Here's how the part is built. I have some questions about the finished solid (model axes, mm). A direction names the side the tool comes from. Round coordinates to 2 decimals unless told otherwise and drop trailing zeros. Order: outer loops, then holes, each group sorted by start corner. A loop starts at its lowest first (then second) coordinate and runs counter-clockwise, first axis right, second up. Notation, with made-up numbers: (-2, 23) - (37, 23) arc R6 ccw to (37, 33) - close; hole circle Ø11 at (31, 3.25). An arc over 180 degrees is marked (long way). One line per item, written item: value.
from build123d import *

# Parameters (mm, degrees)
SKETCH1_R               = 5
BOSS_EXTRUDE1_DEPTH     = 50
SKETCH2_R               = 2
CUT_EXTRUDE1_DEPTH      = 113.087037288
CUT_EXTRUDE3_DEPTH      = 10
CUT_EXTRUDE3_DEPTH_BACK = 10
SKETCH7_W               = 20
SKETCH7_H               = 39.987182744
BOSS_EXTRUDE2_REACH     = 114.087
CUT_EXTRUDE4_REACH      = 114.087
SKETCH9_W               = 20
SKETCH9_H               = 10.896319728
CUT_EXTRUDE6_REACH      = 114.087
SKETCH11_W              = 5
SKETCH11_H              = 3
SKETCH12_W              = 73
SKETCH12_H              = 70
BOSS_EXTRUDE3_DEPTH     = 3
SKETCH13_W              = 6.758772051
SKETCH13_H              = 20
CUT_EXTRUDE7_DEPTH      = 117.122297969
FILLET1_R               = 10


with BuildPart() as part:
    # Sketch1 → Boss-Extrude1 (new body)
    with BuildSketch(Plane.XY):
        with Locations((90.291740814, 26.352640412)):
            Circle(SKETCH1_R)
        Polygon((0, 3), (0, 0), (81.758772051, 0), (91.791740814, 17.924366601), (91.791740814, 23.706854983), (88.791740814, 23.706854983), (88.791740814, 18.706854983), (80, 3), align=None)
    extrude(amount=BOSS_EXTRUDE1_DEPTH)

    # Sketch2 → Cut-Extrude1 (cut, through all)
    with BuildSketch(Plane.XY):
        with Locations((90.291740814, 26.352640412)):
            Circle(SKETCH2_R)
    extrude(amount=CUT_EXTRUDE1_DEPTH, mode=Mode.SUBTRACT)

    # Sketch7 → Cut-Extrude3 (cut, two sides: drawn at the far end of the back side and taken through both)
    with BuildSketch(Plane(origin=(62.254079791, -34.846042362, 0), x_dir=(0, 0, -1), z_dir=(0.8726030546274219, -0.4884300452008377, 0)).offset(-CUT_EXTRUDE3_DEPTH_BACK)):
        with Locations((-25, 59.927032101)):
            Rectangle(SKETCH7_W, SKETCH7_H)
    extrude(amount=CUT_EXTRUDE3_DEPTH + CUT_EXTRUDE3_DEPTH_BACK, mode=Mode.SUBTRACT)

    # Sketch8 → Boss-Extrude2 (add, up to next)
    with BuildSketch(Plane.XY, mode=Mode.PRIVATE) as boss_extrude2_sk1:
        Polygon((66.951015515, 3), (66.951015515, 0), (81.758772051, 0), (79.25400484, 1.667244856), (80, 3), align=None)
    boss_extrude2_tool1 = extrude(boss_extrude2_sk1.sketch, amount=BOSS_EXTRUDE2_REACH, mode=Mode.PRIVATE) - part.part
    add(boss_extrude2_tool1.solids().sort_by_distance((73.552437, 1.463367, 0))[0])

    # Sketch9 → Cut-Extrude4 (cut, up to next)
    with BuildSketch(Plane(origin=(0, 0, 0), x_dir=(0, 0, -1), z_dir=(1, 0, 0)), mode=Mode.PRIVATE) as cut_extrude4_sk1:
        with Locations((-25, 32.01270193)):
            Rectangle(SKETCH9_W, SKETCH9_H)
    cut_extrude4_tool1 = extrude(cut_extrude4_sk1.sketch, amount=CUT_EXTRUDE4_REACH, mode=Mode.PRIVATE) & part.part
    add(cut_extrude4_tool1.solids().sort_by_distance((0, 32.012702, 25))[0], mode=Mode.SUBTRACT)

    # Sketch11 → Cut-Extrude6 (cut, up to next)
    with BuildSketch(Plane.XY.offset(50), mode=Mode.PRIVATE) as cut_extrude6_sk1:
        with Locations((2.5, 1.5)):
            Rectangle(SKETCH11_W, SKETCH11_H)
    cut_extrude6_tool1 = extrude(cut_extrude6_sk1.sketch, amount=-CUT_EXTRUDE6_REACH, mode=Mode.PRIVATE) & part.part
    add(cut_extrude6_tool1.solids().sort_by_distance((2.5, 1.5, 50))[0], mode=Mode.SUBTRACT)

    # Sketch12 → Boss-Extrude3 (add, through all)
    with BuildSketch(Plane(origin=(0, 3, 0), x_dir=(1, 0, 0), z_dir=(0, 1, 0))):
        with Locations((38.5, -25)):
            Rectangle(SKETCH12_W, SKETCH12_H)
    extrude(amount=-BOSS_EXTRUDE3_DEPTH)

    # Sketch13 → Cut-Extrude7 (cut, through all)
    with BuildSketch(Plane(origin=(0, 3, 0), x_dir=(1, 0, 0), z_dir=(0, 1, 0))):
        with Locations((78.379386025, -25)):
            Rectangle(SKETCH13_W, SKETCH13_H)
    extrude(amount=-CUT_EXTRUDE7_DEPTH, mode=Mode.SUBTRACT)

    # Fillet1
    fillet1_edges = [part.edges().sort_by_distance(p)[0] for p in [
        (75, 1.5, -10),
        (2, 1.5, -10),
        (2, 1.5, 60),
        (75, 1.5, 60),
    ]]
    fillet(fillet1_edges, radius=FILLET1_R - 0.0001)  # a hair under: the kernel refuses the full size


solid = part.part
Q1. If we section it at D-D, the plane z = 20: Please give me the cut outline in (x, y), then the cut area to 3 significant figures.
Results list:
outline: (2, 0) - (75, 0) - (75, 3) - (2, 3) - close
area: 219 mm²
Q2. Will these pins go through, and if not, where does the flat tip stop? pin 1 (10 mm diameter, centred on x = 84, z = 19, fed in from +Y); pin 2 (1 mm diameter, centred on x = 23, z = 38.5, fed in from +Y); pin 3 (6.5 mm diameter, centred on x = 90.29, y = 26.35, fed in from +Z).
Results list:
pin 1: y = 30.12
pin 2: y = 3
pin 3: z = 50
Q3. If I drill on line 1 along Y through (x, z) = (72, 36.5); line 2 along X through (y, z) = (18.5, 36); line 3 along X through (y, z) = (25.5, 35.5), over which ranges is the centre line in solid material (lowest first)?
Results list:
line 1: 0 to 3
line 2: 88.68 to 91.79
line 3: 85.36 to 88.48, 92.1 to 95.22
Q4. If we section it at B-B, the plane z = 41.5: Please give me the cut outline in (x, y), then the cut area to 3 significant figures.
Results list:
outline: (2, 0) - (81.76, 0) - (91.79, 17.92) - (91.79, 21.58) arc R5 ccw (long way) to (88.79, 21.58) - (88.79, 18.71) - (80, 3) - (2, 3) - close; hole circle Ø4 at (90.29, 26.35)
area: 370 mm²
Q5. If we section it at A-A, the plane y = 14: Please give me the cut outline in (x, z).
Results list:
outline: (86.16, 0) - (89.6, 0) - (89.6, 15) - (86.16, 15) - close; (86.16, 35) - (89.6, 35) - (89.6, 50) - (86.16, 50) - close
Q6. If we section it at C-C, the plane x = 17.5: Please give me the cut outline in (y, z).
Results list:
outline: (0, -10) - (3, -10) - (3, 60) - (0, 60) - close
Q7. Which directions (+Z, -Z, +X, -X, +Y, -Y) give clear straight access to the entire face, cutting with the end or side of a thin tool? Please do faces 4 (the flat face through (40, 3, 25)), 5 (the flat face through (91.792, 20, 7)), 6 (the flat face through (84.457, 10.963, 7.395)).
Results list:
face 4: +Z, -Z, -X, +Y
face 5: +Z, -Z, +X, -Y
face 6: +Z, -Z, -X
Q8. We'd pull the mould along Z, two halves only. Please class faces 1 (the flat face through (91.792, 20, 42)), 2 (the flat face through (75, 2, 25)), 3 (the cylindrical face through (4.85, 1.48, -6.99)): released by +Z, released by -Z, zero draft, split by the parting line, or undercut.
Results list:
face 1: zero draft
face 2: undercut
face 3: released by -Z
